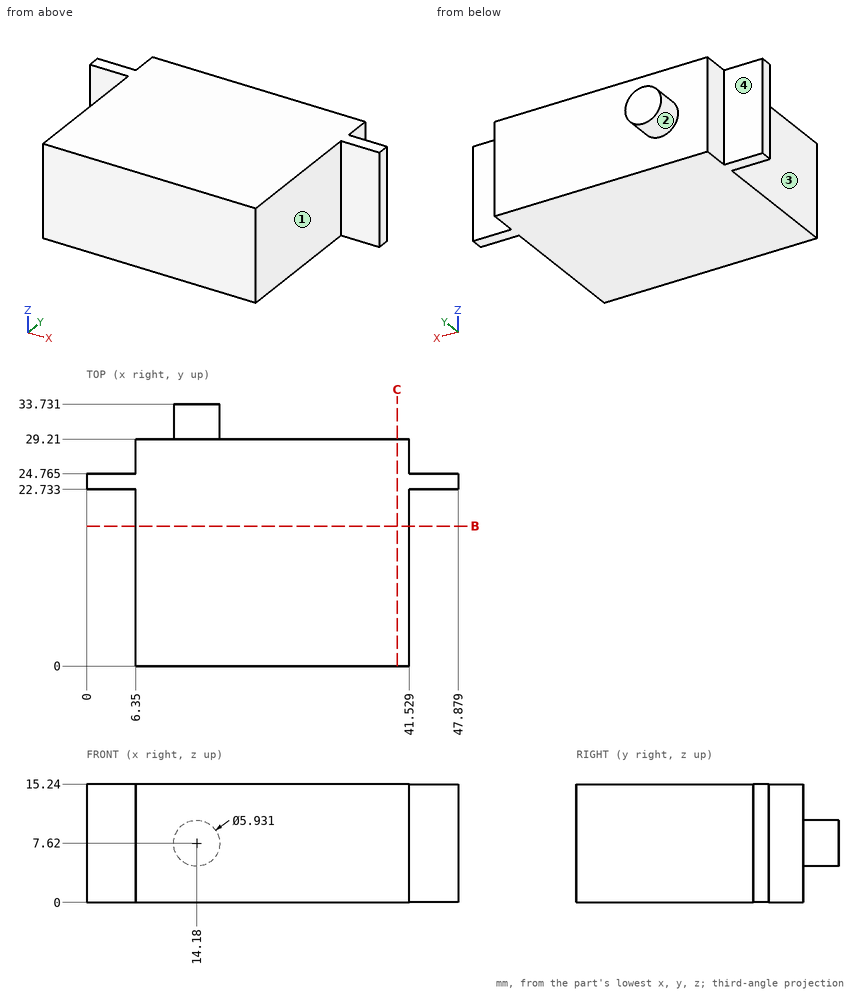
Geometry: see drawing. Coordinates: mm, zero at the bounding-box minimum. A direction names the side the tool comes from. Give positions to 0.01 mm unless a question says otherwise; leave off trailing zeros. Loops run counter-clockwise (first coordinate to the right, second up) from the corner with the lowest first, then second, coordinate; pieces in that order, holes last. Notation, with made-up numbers: M -40,-12 L 16,-12 A11 ccw 16,4 Z; hole C -36.75,-15.5 d11. An arc over 180 degrees is marked long. Use one line per item in the form item = value.
1. Line query: L1, parallel to Y at x = 39, z = 3; L2, parallel to X at y = 10, z = 1; L3, parallel to Y at x = 3, z = 2.5 (1 decimal). Output: solid intervals per line, ascending.
Numbers:
L1 = 0 to 29.21
L2 = 6.35 to 41.53
L3 = 22.7 to 24.8
2. Reachability of the marked faces 1, 2, 3 and 4 from +Z, -Z, +X, -X, +Y, -Y: full face, straight path, thin tool, end or side. Return the list, or none.
Numbers:
face_1 = +Z, -Z, +X, -Y
face_2 = +Y
face_3 = +Z, -Z, -X, -Y
face_4 = +Z, -Z, -X, +Y
3. First-contact query: pin 1 (1.9 mm diameter, centred on x = 46, z = 4, fed in from +Y) (3 decimals); pin 2 (4 mm diameter, centred on y = 7, z = 10.5, fed in from +X); pin 3 (1.5 mm diameter, centred on x = 25, z = 2, fed in from +Y). Flat tips, straight axial feed; report the tip coordinate or a pass-through.
Numbers:
pin_1 = 24.765
pin_2 = 41.53
pin_3 = 29.21
4. Section query C-C, the plane x = 40. Return the cut outline in (y, z), and give its area (3 significant figures).
Numbers:
outline = M 0,0 L 29.21,0 L 29.21,15.24 L 0,15.24 Z
area = 445 mm²
5. Section query B-B, the plane y = 18. Return the cut outline in (x, z).
Numbers:
outline = M 6.35,0 L 41.53,0 L 41.53,15.24 L 6.35,15.24 Z
